The model under review builds one solid part; all positions refer to its coordinate system, in mm. Face numbers are marked on the shaded views. A direction names the side the tool comes from. Round coordinates to 2 decimals unless told otherwise and drop trailing zeros. Write each loop counter-clockwise with the first axis right and the second up, starting at its lowest first coordinate (ties: lowest second). Pieces come first, ordered by that corner, then holes. Notation, with made-up numbers: (66.25, 70.25) - (111.25, 70.25) arc R20 ccw to (111.25, 95.25) - close; hole circle Ø10 at (7.5, 52.5). An arc over 180 degrees is marked (long way). Use one line per item in the form item = value.
from build123d import *

# Parameters (mm, degrees)
F0_R     = 11.25
F1_DEPTH = 4.5
F2_R     = 10.25
F3_DEPTH = 1
F4_R     = 15.75
F5_DEPTH = 1.5
F7_DEPTH = 5
F8_R     = 0.5


with BuildPart() as f1:
    # F0 (on Front) → F1 (new body)
    with BuildSketch(Plane.XZ):
        Circle(F0_R)
    extrude(amount=F1_DEPTH)

    # F2 (on face) → F3 (join)
    with BuildSketch(Plane(origin=(0, 0, 0), x_dir=(-1, 0, 0), z_dir=(0, 1, 0))):
        Circle(F2_R)
    extrude(amount=F3_DEPTH)

    # F4 (on face) → F5 (join)
    with BuildSketch(Plane(origin=(0, 1, 0), x_dir=(-1, 0, 0), z_dir=(0, 1, 0))):
        Circle(F4_R)
    extrude(amount=F5_DEPTH)

    # F6 (on face) → F7 (cut)
    with BuildSketch(Plane(origin=(0, 2.5, 0), x_dir=(-1, 0, 0), z_dir=(0, 1, 0))):
        Polygon((4.875, 8.4437476869), (-4.875, 8.4437476869), (-9.75, 0), (-4.875, -8.4437476869), (4.875, -8.4437476869), (9.75, 0), align=None)
    extrude(amount=-F7_DEPTH, mode=Mode.SUBTRACT)

    # F8
    f8_edges = [f1.edges().sort_by_distance(p)[0] for p in [
        (15.75, 2.5, 0),
        (0, 2.5, 8.443748),
        (7.3125, 2.5, 4.221874),
        (7.3125, 2.5, -4.221874),
        (0, 2.5, -8.443748),
        (-7.3125, 2.5, -4.221874),
        (-7.3125, 2.5, 4.221874),
    ]]
    fillet(f8_edges, radius=F8_R)


solid = f1.part
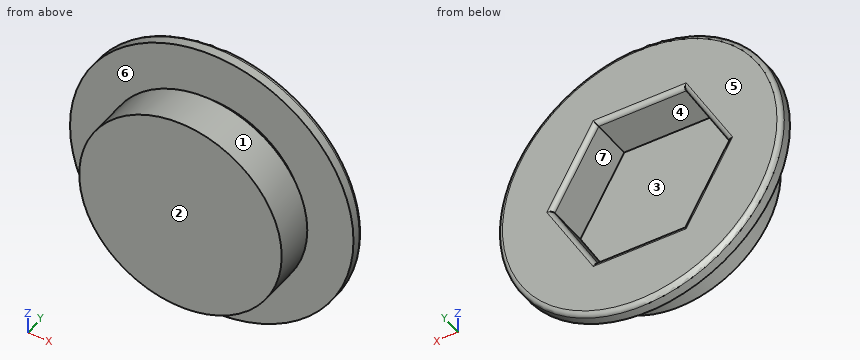
(1) Machinability: for the marked faces 5, 6 and 7, which of the approach directions +Z, -Z, +X, -X, +Y, -Y give a long, thin tool a straight path to every point of the face, cutting with its end or side? Answer none if there is none.
Geometry results:
face_5 = +Z, -Z, +X, -X, +Y
face_6 = none
face_7 = +Y
(2) The part is to be moulded in two halves that separate along Z. For the marked faces 1, 2, 3 and 4, say which applies: +Z half, -Z half, draft (parallel to the pull), parting line (faces both ways), or undercut.
Geometry results:
face_1 = parting line
face_2 = draft
face_3 = undercut
face_4 = undercut
(3) Insertion check: P1, Ø3.5, axis at x = -2, y = 0.5, coming from the +Z side; P2, Ø3, axis at y = 0.5, z = 3.5, coming from the -X side; P3, Ø3, axis at y = 0, z = -8.5, coming from the +X side; P4, Ø2, axis at y = -1, z = -12.5, coming from the -X side. Each pin has a flat end and moves straight along its axis. Give the tip position at first contact, or say it passes through.
Geometry results:
P1 = 15.75
P2 = -15.61
P3 = 13.91
P4 = through
(4) Add section B-B on x = 0. Write out the cut boundary in (y, z), then the cut area to 3 significant figures.
Geometry results:
outline = (-4.5, -11.25) - (0, -11.25) - (0, -10.25) - (1, -10.25) - (1, -15.75) - (2, -15.75) arc R0.5 ccw to (2.5, -15.25) - (2.5, -8.94) arc R0.5 ccw to (2, -8.44) - (-2.5, -8.44) - (-2.5, 8.44) - (2, 8.44) arc R0.5 ccw to (2.5, 8.94) - (2.5, 15.25) arc R0.5 ccw to (2, 15.75) - (1, 15.75) - (1, 10.25) - (0, 10.25) - (0, 11.25) - (-4.5, 11.25) - close
area = 84.3 mm2
(5) Add section C-C on y = -1. Write out the cut boundary in (x, z) (3 decimals), then the cut area to 3 significant figures.
Geometry results:
outline = circle Ø22.5 at (0, 0); hole (-9.75, 0) - (-4.875, -8.444) - (4.875, -8.444) - (9.75, 0) - (4.875, 8.444) - (-4.875, 8.444) - close
area = 151 mm2
(6) Add section A-A on y = 1.5. Write out the cut boundary in (x, z) (3 decimals), then the cut area to 3 significant figures.
Geometry results:
outline = circle Ø31.5 at (0, 0); hole (-9.75, 0) - (-4.875, -8.444) - (4.875, -8.444) - (9.75, 0) - (4.875, 8.444) - (-4.875, 8.444) - close
area = 532 mm2
(7) To check wall thickness, follow L1, parallel to Y at x = 3, z = 10; L2, parallel to Y at x = 9, z = -11.5; L3, parallel to Z at x = 9, y = -0.25. State the ranges of each line that lie inside material, in increasing order.
Geometry results:
L1 = -4.5 to 0, 1 to 2.5
L2 = 1 to 2.5
L3 = -6.75 to -1.3, 1.3 to 6.75
